Solid Edge part; units mm, degrees
sketch "Sketch1" plane through (0, 0, 0) normal (1, 0, 0) x (0, 1, 0)
  line L0 (-37.6609, -235.0291) -> (52.3391, -79.1445)
  line L1 (17.698, -79.1445) -> (52.3391, -79.1445)
  line L2 (17.698, -79.1445) -> (-72.302, -235.0291)
  line L3 (-72.302, -235.0291) -> (-37.6609, -235.0291)
  dimension "D1" = 37.6609
extrude "Protrusion1" add sketch "Sketch1" against normal blind 3
sketch "Sketch2" plane through (0, -21.8205, 20.1807) normal (1, 0, 0) x (0, 1, 0)
  circle A0 centre (50.5934, -110.1432) radius 5
  circle A1 centre (-1.4066, -200.2098) radius 5
extrude "ExtrudedProtrusion_2" add sketch "Sketch2" along normal blind 11
mirror "Mirror1" about plane through (5, -21.8205, 20.1506) normal (1, 0, 0) of "Protrusion1"
sketch "Sketch3" plane through (11.5, -54.9814, -235.0291) normal (0, 0, -1) x (0, 1, 0)
  line L0 (-28.8857, -24.7239) -> (39.7131, -24.7239)
  line L1 (39.7131, -24.7239) -> (39.7131, 10.9355)
  line L2 (39.7131, 10.9355) -> (-28.8857, 10.9355)
  line L3 (-28.8857, 10.9355) -> (-28.8857, -24.7239)
extrude "ExtrudedProtrusion_13" add sketch "Sketch3" along normal blind 5
properties material "Aluminum, 6061-T6"
Build history of the part. All positions in model axes, mm. A direction names the side the tool comes from. Round coordinates to 2 decimals unless told otherwise and drop trailing zeros. Write each loop counter-clockwise with the first axis right and the second up, starting at its lowest first coordinate (ties: lowest second). Pieces come first, ordered by that corner, then holes. Notation, with made-up numbers: (2, -9) - (31, -9) arc R23 ccw to (31, 15) - close; hole circle Ø9 at (8.5, 12.25). An arc over 180 degrees is marked (long way). Use CSV: the item, a comma, the result in double quotes.
(1) Wall check: line 1 (X direction, y = -1.5, z = -139); line 2 (Z direction, x = -6, y = -36); line 3 (Z direction, x = 10.5, y = -30). Give the ranges that are in metal, low to high.
Response:
line 1,"-3 to 0, 10 to 13"
line 2,"-240.03 to -235.03"
line 3,"-240.03 to -235.03, -221.76 to -161.76"
(2) Band-saw the part on C-C (z = -156.5). Write the cut outline in (x, y).
Response:
outline,"(-3, -26.96) - (0, -26.96) - (0, 7.68) - (-3, 7.68) - close; (10, -26.96) - (13, -26.96) - (13, 7.68) - (10, 7.68) - close"
(3) Mould opens along Z. For faces 1 (the flat face through (-1.479, -26.672, -155.996)), 2 (the flat face through (5, -49, -240.029)), 3 (the flat face through (11.479, 7.969, -155.996)), 4 (the flat face through (-13.224, -50, -237)) say: pulls with the +Z half, pulls with the -Z half, needs draft (parallel to the pull), parting line crosses it, or undercut.
Response:
face 1,"pulls with the +Z half"
face 2,"pulls with the -Z half"
face 3,"undercut"
face 4,"needs draft"
(4) Band-saw the part on B-B (y = -8). Write the cut outline in (x, z), plus the area to 3 significant figures.
Response:
outline,"(-3, -183.65) - (0, -183.65) - (0, -123.65) - (-3, -123.65) - close; (10, -183.65) - (13, -183.65) - (13, -123.65) - (10, -123.65) - close"
area,"360 mm²"
(5) 3-axis set-ups, long thin cutter, end or side, ignore diameter. For faces 5 (the flat face through (-1.48, 6.71, -158.18)), 6 (the flat face through (13, -15, -157)), 7 (the flat face through (-3, -15, -157)), 8 (the cylindrical face through (4.93, 31.46, -94.18)), 9 (the flat face through (11.479, -27.932, -158.178)): which of +Z, -Z, +X, -X, +Y, -Y reach the whole face in a straight line?
Response:
face 5,"+X, -X, +Y"
face 6,"+Z, +X, +Y, -Y"
face 7,"+Z, -X, +Y, -Y"
face 8,"none"
face 9,"+Z, +X, -X, -Y"
(6) Band-saw the part on A-A (y = -33). Write the cut outline in (x, z), plus the area to 3 significant figures.
Response:
outline,"(-13.22, -240.03) - (22.44, -240.03) - (22.44, -235.03) - (-13.22, -235.03) - close; (-3, -226.96) - (0, -226.96) - (0, -166.96) - (-3, -166.96) - close; (10, -226.96) - (13, -226.96) - (13, -166.96) - (10, -166.96) - close"
area,"538 mm²"
(7) Pin check, flat tips, straight feed: P1, Ø12, axis at x = 17, z = -125, coming from the +Y side; P2, Ø1.5, axis at x = 4, z = -237, coming from the +Y side; P3, Ø4, axis at x = 1, z = -182, coming from the +Y side. Stop position of each tip, or through.
Response:
P1,"y = 28.45"
P2,"y = -15.27"
P3,"y = -6.04"
(8) Band-saw the part on D-D (y = -57). Write the cut outline in (x, z), plus the area to 3 significant figures.
Response:
outline,"(-13.22, -240.03) - (22.44, -240.03) - (22.44, -235.03) - (13, -235.03) - (13, -208.53) - (10, -208.53) - (10, -235.03) - (0, -235.03) - (0, -208.53) - (-3, -208.53) - (-3, -235.03) - (-13.22, -235.03) - close"
area,"337 mm²"
